```python
from build123d import *

# Parameters (mm, degrees)
SKETCH_1_R          = 1
SKETCH_1_R_2        = 5.5
EXTRUDE_1_DEPTH     = 2
EXTRUDE_2_DEPTH     = 20
EXTRUDE_3_DEPTH     = 20
SKETCH_6_W          = 15
SKETCH_6_H          = 20
EXTRUDE_9_DEPTH     = 4
EXTRUDE_10_DEPTH    = 5
EXTRUDE_11_DEPTH    = 5
CUT_EXTRUDE_3_DEPTH = 10
SKETCH_11_R         = 3
CUT_EXTRUDE_4_DEPTH = 2


with BuildPart() as part:
    # Sketch 1 → Extrude 1 (new body)
    with BuildSketch(Plane.XY):
        with BuildLine():
            ThreePointArc((-8.3498366, -12.037658774), (0, -9.8003268), (8.3498366, -12.037658774))
            Line((8.3498366, -12.037658774), (12.871581666, -14.648289505))
            ThreePointArc((12.871581666, -14.648289505), (16.887495374, -9.75), (19.121581666, -3.822971957))
            Line((19.121581666, -3.822971957), (14.5998366, -1.212341226))
            ThreePointArc((14.5998366, -1.212341226), (8.487331974, 4.9001634), (6.25, 13.25))
            Line((6.25, 13.25), (6.25, 18.471261462))
            ThreePointArc((6.25, 18.471261462), (0, 19.5), (-6.25, 18.471261462))
            Line((-6.25, 18.471261462), (-6.25, 13.25))
            ThreePointArc((-6.25, 13.25), (-8.487331974, 4.9001634), (-14.5998366, -1.212341226))
            Line((-14.5998366, -1.212341226), (-19.121581666, -3.822971957))
            ThreePointArc((-19.121581666, -3.822971957), (-16.887495374, -9.75), (-12.871581666, -14.648289505))
            Line((-12.871581666, -14.648289505), (-8.3498366, -12.037658774))
        make_face()
        with Locations((-11.4748366, -6.625)):
            Circle(SKETCH_1_R, mode=Mode.SUBTRACT)
        with Locations((11.4748366, -6.625)):
            Circle(SKETCH_1_R, mode=Mode.SUBTRACT)
        Circle(SKETCH_1_R_2, mode=Mode.SUBTRACT)
        with Locations((0, 13.25)):
            Circle(SKETCH_1_R, mode=Mode.SUBTRACT)
    extrude(amount=EXTRUDE_1_DEPTH)

    # Sketch 1_3 → Extrude 2 (add)
    with BuildSketch(Plane.XY):
        with BuildLine():
            Line((6.55834649, -15.140610665), (5.773502692, -16.5))
            Line((5.773502692, -16.5), (10.392304845, -16.5))
            ThreePointArc((10.392304845, -16.5), (0, 19.5), (-10.392304845, -16.5))
            Line((-10.392304845, -16.5), (-5.773502692, -16.5))
            Line((-5.773502692, -16.5), (-6.55834649, -15.140610665))
            ThreePointArc((-6.55834649, -15.140610665), (0, 16.5), (6.55834649, -15.140610665))
        make_face()
    extrude(amount=-EXTRUDE_2_DEPTH)

    # Sketch 1_4 → Extrude 3 (add)
    with BuildSketch(Plane.XY):
        with BuildLine():
            Line((5.773502692, -16.5), (6.55834649, -15.140610665))
            ThreePointArc((6.55834649, -15.140610665), (3.348874738, -16.156578783), (0, -16.5))
            Line((0, -16.5), (5.773502692, -16.5))
        make_face()
        with BuildLine():
            Line((10.392304845, -16.5), (5.773502692, -16.5))
            Line((5.773502692, -16.5), (4.321384636, -19.015142251))
            ThreePointArc((4.321384636, -19.015142251), (7.463554761, -18.015142251), (10.392304845, -16.5))
        make_face()
        with BuildLine():
            Line((4.321384636, -19.015142251), (5.773502692, -16.5))
            Line((5.773502692, -16.5), (0, -16.5))
            Line((0, -16.5), (-5.773502692, -16.5))
            Line((-5.773502692, -16.5), (-4.321384636, -19.015142251))
            ThreePointArc((-4.321384636, -19.015142251), (0, -19.5), (4.321384636, -19.015142251))
        make_face()
        with BuildLine():
            ThreePointArc((0, -16.5), (-3.348874738, -16.156578783), (-6.55834649, -15.140610665))
            Line((-6.55834649, -15.140610665), (-5.773502692, -16.5))
            Line((-5.773502692, -16.5), (0, -16.5))
        make_face()
        with BuildLine():
            Line((-4.321384636, -19.015142251), (-5.773502692, -16.5))
            Line((-5.773502692, -16.5), (-10.392304845, -16.5))
            ThreePointArc((-10.392304845, -16.5), (-7.463554761, -18.015142251), (-4.321384636, -19.015142251))
        make_face()
    extrude(amount=-EXTRUDE_3_DEPTH)

    # Sketch 6 → Extrude 9 (add)
    with BuildSketch(Plane(origin=(0, -14.648289505, 0), x_dir=(1, 0, 0), z_dir=(0, 1, 0))):
        with Locations((20.371581666, 10)):
            Rectangle(SKETCH_6_W, SKETCH_6_H)
        with Locations((-20.371581666, 10)):
            Rectangle(SKETCH_6_W, SKETCH_6_H)
    extrude(amount=EXTRUDE_9_DEPTH)

    # Sketch 8 → Extrude 10 (add)
    with BuildSketch(Plane(origin=(0, 0, -20), x_dir=(-1, 0, 0), z_dir=(0, 0, -1))):
        with BuildLine():
            Line((-17.172554049, 9.238689703), (-27.871581666, -10.648289505))
            Line((-27.871581666, -10.648289505), (-16.335970452, -10.648289505))
            ThreePointArc((-16.335970452, -10.648289505), (-19.48276903, -0.819579727), (-17.172554049, 9.238689703))
        make_face()
    extrude(amount=-EXTRUDE_10_DEPTH)

    # Sketch 8_3 → Extrude 11 (add)
    with BuildSketch(Plane(origin=(0, 0, -20), x_dir=(-1, 0, 0), z_dir=(0, 0, -1))):
        with BuildLine():
            Line((27.871581666, -10.648289505), (17.172554049, 9.238689703))
            ThreePointArc((17.172554049, 9.238689703), (19.48276903, -0.819579727), (16.335970452, -10.648289505))
            Line((16.335970452, -10.648289505), (27.871581666, -10.648289505))
        make_face()
    extrude(amount=-EXTRUDE_11_DEPTH)

    # Sketch 9 → Cut-Extrude 3 (cut)
    with BuildSketch(Plane(origin=(0, -10.648289505, 0), x_dir=(1, 0, 0), z_dir=(0, 1, 0))):
        with BuildLine():
            ThreePointArc((-25.5, 7.5), (-24, 6), (-22.5, 7.5))
            Line((-22.5, 7.5), (-25.5, 7.5))
        make_face()
        with BuildLine():
            Line((-25.5, 7.5), (-22.5, 7.5))
            ThreePointArc((-22.5, 7.5), (-24, 9), (-25.5, 7.5))
        make_face()
        with BuildLine():
            ThreePointArc((22.5, 7.5), (24, 6), (25.5, 7.5))
            Line((25.5, 7.5), (24, 7.5))
            Line((24, 7.5), (22.5, 7.5))
        make_face()
        with BuildLine():
            Line((24, 7.5), (25.5, 7.5))
            ThreePointArc((25.5, 7.5), (24, 9), (22.5, 7.5))
            Line((22.5, 7.5), (24, 7.5))
        make_face()
    extrude(amount=-CUT_EXTRUDE_3_DEPTH, mode=Mode.SUBTRACT)

    # Sketch 11 → Cut-Extrude 4 (cut)
    with BuildSketch(Plane(origin=(0, -10.648289505, 0), x_dir=(1, 0, 0), z_dir=(0, 1, 0))):
        with Locations((-24, 7.5)):
            Circle(SKETCH_11_R)
        with Locations((24, 7.5)):
            Circle(SKETCH_11_R)
    extrude(amount=-CUT_EXTRUDE_4_DEPTH, mode=Mode.SUBTRACT)


solid = part.part
```
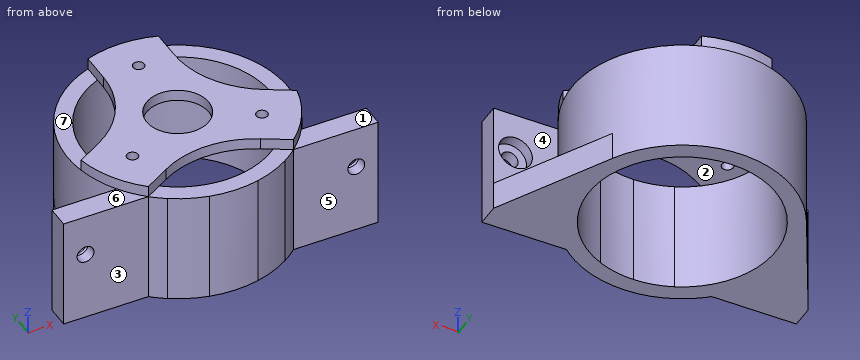
Could you check a few things on this model? Use its own coordinates, in mm. Face numbers are marked on the shaded views. A direction names the side the tool comes from. Round coordinates to 2 decimals unless told otherwise and drop trailing zeros. Loops run counter-clockwise (first coordinate to the right, second up) from the corner with the lowest first, then second, coordinate; pieces in that order, holes last. Notation, with made-up numbers: (0, 29) - (29, 29) arc R16 ccw to (29, 34) - close; hole circle Ø10 at (62.5, 22). An arc over 180 degrees is marked (long way). Answer in a Markdown table with one row per item. Add a question column.
(1) If we section it at B-B (z = -17.75): Please give me the cut outline in (x, y), plus the area to 3 significant figures.
(2) For the marked faces 5, 6 and 7, which set-ups out of +Z, -Z, +X, -X, +Y, -Y let a thin tool reach every point of the face, with its end or its side?
(3) If we section it at D-D (y = 8): Please give me the cut outline in (x, z), plus the area to 3 significant figures.
(4) I need wall thicknesses on line 1 along X through (y, z) = (-11.9, -7.5); line 2 along Y through (x, z) = (-14.5, -2); line 3 along Y through (x, z) = (4, -13). Which ranges of each line are inside material? Lowest first, please.
(5) I'm going to push flat-ended pins straight in: pin 1 (5 mm diameter, centred on x = 24, z = -7.5, fed in from -Y); pin 2 (12 mm diameter, centred on x = 8, z = -9.5, fed in from -Y); pin 3 (5 mm diameter, centred on y = -2, z = -0.5, fed in from -X). Where does each tip first touch, or does it pass through?
(6) If we section it at C-C (x = 24): Please give me the cut outline in (y, z).
(7) If we mould it in two halves opening along Y, with no side actions, what happens to the marked faces 1, 2, 3 and 4? For each: pulls with the +Y half, pulls with the -Y half, needs draft (parallel to the pull), parting line crosses it, or undercut.
(8) If we section it at A-A (z = -7.5): Please give me the cut outline in (x, y), plus the area to 3 significant figures.
Model answer:
| question | item | result |
|---|---|---|
| 1 | outline | (-27.87, -14.65) - (-12.87, -14.65) arc R19.5 ccw to (12.87, -14.65) - (27.87, -14.65) - (27.87, -10.65) - (17.17, 9.24) arc R19.5 ccw to (-17.17, 9.24) - (-27.87, -10.65) - close; hole circle Ø33 at (0, 0) |
| 1 | area | 600 mm² |
| 2 | face 5 | +Z, -Z, +X, -Y |
| 2 | face 6 | +Z, -X, -Y |
| 2 | face 7 | +Z, -X, +Y |
| 3 | outline | (-17.84, -20) - (-14.43, -20) - (-14.43, 0) - (-17.78, 0) - (-17.78, -15) - (-17.84, -15) - close; (-7.1, 0) - (7.1, 0) - (7.1, 2) - (-7.1, 2) - close; (14.43, -20) - (17.84, -20) - (17.84, -15) - (17.78, -15) - (17.78, 0) - (14.43, 0) - close |
| 3 | area | 163 mm² |
| 4 | line 1 | x = -27.87 to -27, -21 to -11.43, 11.43 to 21, 27 to 27.87 |
| 4 | line 2 | y = -14.65 to -7.87, 7.87 to 13.04 |
| 4 | line 3 | y = -19.09 to -16.01, 16.01 to 19.09 |
| 5 | pin 1 | stops at y = -14.65 |
| 5 | pin 2 | stops at y = -19.4 |
| 5 | pin 3 | stops at x = -19.5 |
| 6 | outline | (-14.65, -20) - (-3.45, -20) - (-3.45, -15) - (-10.65, -15) - (-10.65, -10.5) - (-12.65, -10.5) - (-12.65, -9) - (-14.65, -9) - close; (-14.65, -6) - (-12.65, -6) - (-12.65, -4.5) - (-10.65, -4.5) - (-10.65, 0) - (-14.65, 0) - close |
| 7 | face 1 | needs draft |
| 7 | face 2 | undercut |
| 7 | face 3 | pulls with the -Y half |
| 7 | face 4 | undercut |
| 8 | outline | (-27.87, -14.65) - (-25.5, -14.65) - (-25.5, -12.65) - (-27, -12.65) - (-27, -10.65) - (-27.87, -10.65) - close; (-22.5, -14.65) - (-12.87, -14.65) arc R19.5 ccw to (12.87, -14.65) - (22.5, -14.65) - (22.5, -12.65) - (21, -12.65) - (21, -10.65) - (16.34, -10.65) arc R19.5 ccw (long way) to (-16.34, -10.65) - (-21, -10.65) - (-21, -12.65) - (-22.5, -12.65) - close; (25.5, -14.65) - (27.87, -14.65) - (27.87, -10.65) - (27, -10.65) - (27, -12.65) - (25.5, -12.65) - close; hole circle Ø33 at (0, 0) |
| 8 | area | 408 mm² |
